Part model, mm, in its own coordinate system. Face numbers are marked on the shaded views. Coordinates: 2 decimals unless noted, no trailing zeros. Write each loop counter-clockwise with the first axis right and the second up, starting at its lowest first coordinate (ties: lowest second). Pieces come first, ordered by that corner, then holes. Notation, with made-up numbers: (41.25, 38.25) -> (93.25, 38.25) arc R32 ccw to (93.25, 64.25) -> close; hole circle Ø7 at (49.25, 43). An arc over 180 degrees is marked (long way). Write item = value, one per line.
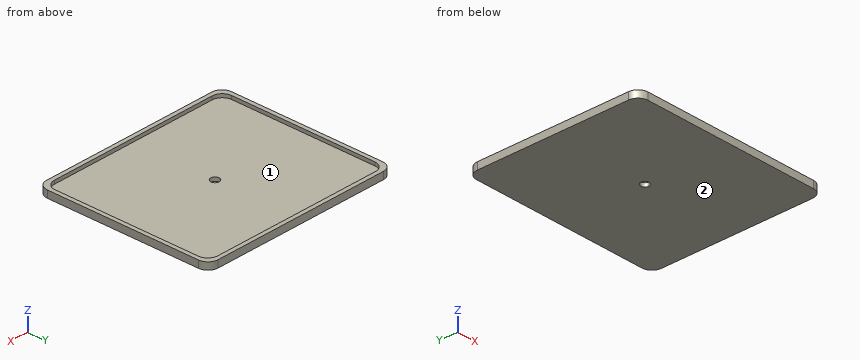
from build123d import *

# Parameters (mm, degrees)
F1_DEPTH = 1.8
F2_R     = 5
F3_DEPTH = 3.5
F4_R     = 5
F5_R     = 5


# Not quite as in the source:
# - a feature names something its author has since deleted; it is built from what else it names


with BuildPart() as f1:
    # F0 (on Top) → F1 (new body)
    with BuildSketch(Plane.XY):
        Polygon((-98, 0), (0, 0), (0, 85), (-49, 85), (-98, 85), align=None)
        Polygon((-96, 83), (-49, 83), (-2, 83), (-2, 2), (-96, 2), align=None, mode=Mode.SUBTRACT)
        Polygon((-2, 83), (-49, 83), (-96, 83), (-96, 2), (-2, 2), align=None)
        with BuildLine():
            ThreePointArc((-46.9, 42.5), (-50.4849242405, 41.0150757595), (-49, 44.6))
            ThreePointArc((-49, 44.6), (-47.5150757595, 43.9849242405), (-46.9, 42.5))
        make_face(mode=Mode.SUBTRACT)
    extrude(amount=F1_DEPTH)

    # F2
    f2_edges = [f1.edges().sort_by_distance(p)[0] for p in [
        (-98, 85, 0.9),
        (-98, 0, 0.9),
        (0, 0, 0.9),
        (0, 85, 0.9),
    ]]
    fillet(f2_edges, radius=F2_R)

    # F0 (on Top) → F3 (join)
    with BuildSketch(Plane.XY):
        Polygon((-98, 0), (0, 0), (0, 85), (-49, 85), (-98, 85), align=None)
        Polygon((-96, 83), (-49, 83), (-2, 83), (-2, 2), (-96, 2), align=None, mode=Mode.SUBTRACT)
    extrude(amount=F3_DEPTH)

    # F4
    f4_edges = [f1.edges().sort_by_distance(p)[0] for p in [
        (0, 85, 1.75),
        (0, 0, 1.75),
        (-98, 0, 1.75),
        (-98, 85, 1.75),
    ]]
    fillet(f4_edges, radius=F4_R)

    # F5
    f5_edges = [f1.edges().sort_by_distance(p)[0] for p in [
        (-96, 83, 2.65),
        (-96, 2, 2.65),
        (-2, 83, 2.65),
        (-2, 2, 2.65),
    ]]
    fillet(f5_edges, radius=F5_R)


solid = f1.part
Q1. Pin check, flat tip, straight feed: pin 1 (1 mm diameter, centred on x = -15.5, y = 32.5, fed in from +Z). Stop position of the tip, or through.
Model answer:
pin_1 = 1.8
Q2. Mould opens along X. For the marked faces 1 and 2 say: released by +X, released by -X, zero draft, split by the parting line, or undercut.
Model answer:
face_1 = undercut
face_2 = zero draft
Q3. Probe line 1 (Y direction, x = -49, z = 1); line 2 (Y direction, x = -28.5, z = 2.6); line 3 (X direction, y = 74.5, z = 3.1). List the from-to ranges inside material, lowest first. Write a range as from..to.
Model answer:
line_1 = 0..40.4, 44.6..85
line_2 = 0..2, 83..85
line_3 = -98..-96, -2..0
Q4. Saw through at B-B on y = 49.5. Give the cut face in (x, z), and give its area (3 significant figures).
Model answer:
outline = (-98, 0) -> (0, 0) -> (0, 3.5) -> (-2, 3.5) -> (-2, 1.8) -> (-96, 1.8) -> (-96, 3.5) -> (-98, 3.5) -> close
area = 183 mm²
Q5. Saw through at A-A on x = -25. Give the cut face in (y, z), and give its area (3 significant figures).
Model answer:
outline = (0, 0) -> (85, 0) -> (85, 3.5) -> (83, 3.5) -> (83, 1.8) -> (2, 1.8) -> (2, 3.5) -> (0, 3.5) -> close
area = 160 mm²
